Input: dimensioned drawing with shaded views. Units: mm. Origin: part minimum x, y, z. Give positions to 0.01 mm unless a question says otherwise; leave off trailing zeros. Write each loop counter-clockwise with the first axis right and the second up, starting at its lowest first coordinate (ties: lowest second). Pieces come first, ordered by that corner, then holes.
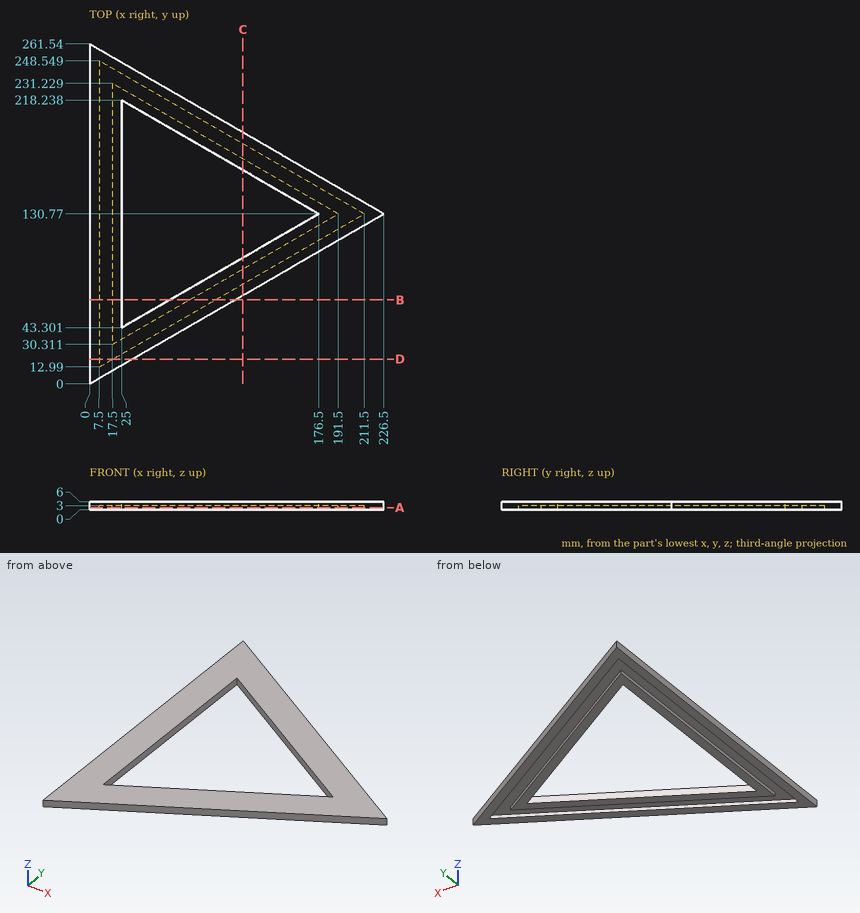
Item 1: Section A-A (z = 1.5). Return loops of the section in (x, y).
Item 2: Ray query, line 1 (X direction, y = 221, z = 1) (1 decimal); line 2 (Y direction, x = 112.5, z = 2.5); line 3 (X direction, y = 35.5, z = 2.5) (1 decimal). Return the intervals inside material, ascending.
Item 3: Section D-D (y = 19). Return loops of the section in (x, z), and give its area (3 significant figures).
Item 4: Section C-C (x = 118). Return loops of the section in (y, z) (1 decimal).
Item 5: Section B-B (y = 64.5). Return loops of the section in (x, z).
Item 6: Pin query (flat end, axial travel): pin 1 (1.5 mm diameter, centred on x = 138.5, z = 1.5, fed in from +Y); pin 2 (1.5 mm diameter, centred on x = 101, z = 4.5, fed in from +Y); pin 3 (3.5 mm diameter, centred on y = 114, z = 2, fed in from +X) (1 decimal). Return the tip coordinate at first contact, or that it passes through.
Solved:
1. outline: (0, 0) - (226.5, 130.77) - (0, 261.54) - close; (17.5, 30.31) - (191.5, 130.77) - (17.5, 231.23) - close; hole (7.5, 12.99) - (211.5, 130.77) - (7.5, 248.55) - close; hole (25, 43.3) - (176.5, 130.77) - (25, 218.24) - close
2. line 1: x = 0 to 7.5, 17.5 to 35.2, 55.2 to 70.2
2. line 2: y = 64.95 to 73.61, 85.16 to 93.82, 167.72 to 176.38, 187.93 to 196.59
2. line 3: x = 0 to 7.5, 17.5 to 26.5, 46.5 to 61.5
3. outline: (0, 0) - (7.5, 0) - (7.5, 3) - (17.91, 3) - (17.91, 0) - (32.91, 0) - (32.91, 6) - (0, 6) - close
3. area: 166 mm2
4. outline: (68.1, 0) - (76.8, 0) - (76.8, 3) - (88.3, 3) - (88.3, 0) - (97, 0) - (97, 6) - (68.1, 6) - close; (164.5, 0) - (173.2, 0) - (173.2, 3) - (184.8, 3) - (184.8, 0) - (193.4, 0) - (193.4, 6) - (164.5, 6) - close
5. outline: (0, 0) - (7.5, 0) - (7.5, 3) - (17.5, 3) - (17.5, 0) - (25, 0) - (25, 6) - (0, 6) - close; (61.72, 0) - (76.72, 0) - (76.72, 3) - (96.72, 3) - (96.72, 0) - (111.72, 0) - (111.72, 6) - (61.72, 6) - close
6. pin 1: stops at y = 182.01
6. pin 2: stops at y = 203.66
6. pin 3: stops at x = 200.5
